Verification items for this drawing (mm, ordinates from the low corner). A direction names the side the tool comes from. Coordinates: 2 decimals unless noted, no trailing zeros. Order: outer loops, then holes, each group sorted by start corner. A loop starts at its lowest first (then second) coordinate and runs counter-clockwise, first axis right, second up.
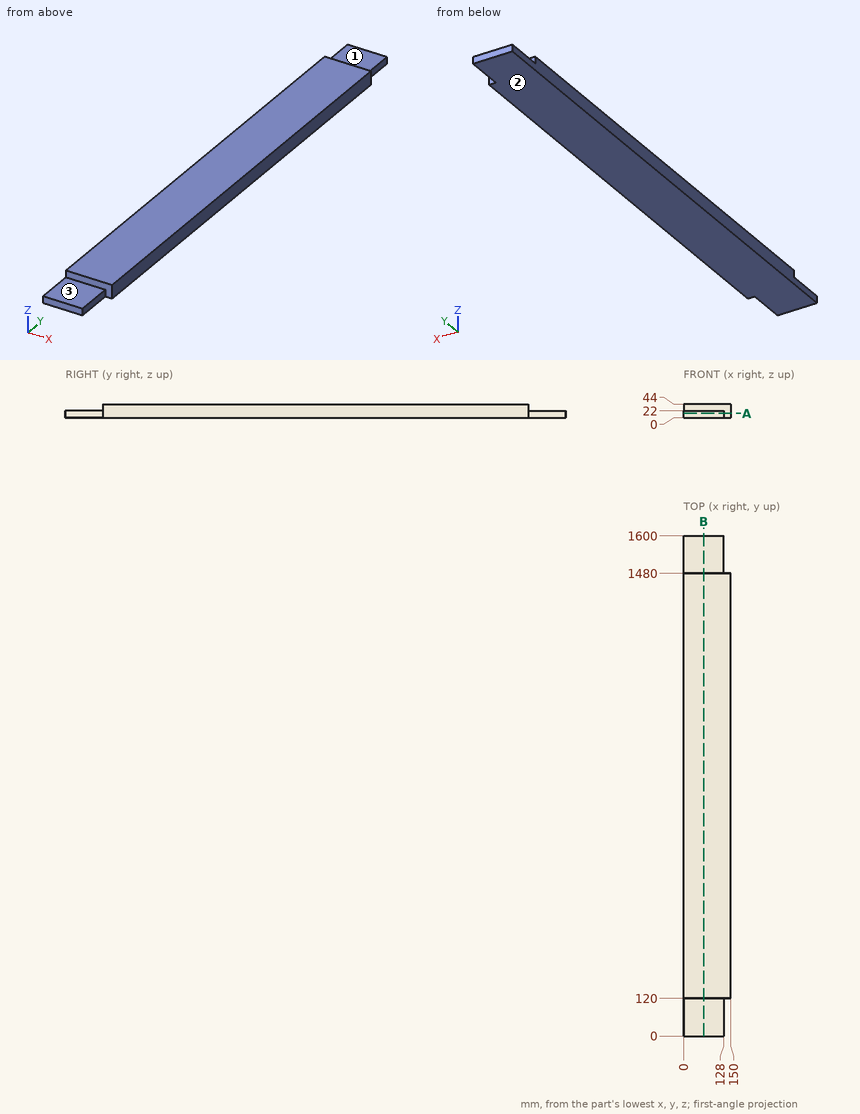
(1) Cross-section at A-A (z = 14). Enter the section's corners in (x, y), and give its area (3 significant figures).
Filled in:
outline: (0, 0) - (128, 0) - (128, 120) - (150, 120) - (150, 1480) - (128, 1480) - (128, 1600) - (0, 1600) - close
area: 235,000 mm2
(2) Cross-section at B-B (x = 64). Enter the section's corners in (y, z), and give its area (3 significant figures).
Filled in:
outline: (0, 0) - (1600, 0) - (1600, 22) - (1480, 22) - (1480, 44) - (120, 44) - (120, 22) - (0, 22) - close
area: 65,100 mm2
(3) Thickness scan on probe 1 along Y at (x, z) = (104, 39). Record the ranges inside material, lowest first.
Filled in:
probe 1: y = 120 to 1480
(4) Go/stop test with flat-tipped pins: P1, Ø6.5, axis at y = 1513.5, z = 16.5, coming from the +X side; P2, Ø5, axis at x = 39.5, z = 36.5, coming from the +Y side. Record where each tip stops, or that it passes through.
Filled in:
P1: stops at x = 128
P2: stops at y = 1480
(5) Tool access check on the marked faces 1, 2 and 3. Record the directions out of +Z, -Z, +X, -X, +Y, -Y that give a thin tool (end or side, any length) a straight path to the whole face; none if there is none.
Filled in:
face 1: +Z, +X, -X, +Y
face 2: -Z, +X, -X, +Y, -Y
face 3: +Z, +X, -X, -Y
